Part print with two shaded views. Sizes in mm from the minimum x, y, z corner. A direction names the side the tool comes from. Round coordinates to 2 decimals unless told otherwise and drop trailing zeros. Order: outer loops, then holes, each group sorted by start corner. A loop starts at its lowest first (then second) coordinate and runs counter-clockwise, first axis right, second up. Notation, with made-up numbers: (8.25, -39) -> (30.25, -39) arc R30 ccw to (30.25, -15) -> close; hole circle Ø4 at (85.5, 72). An arc over 180 degrees is marked (long way). Use a Markdown table: item, result. Add a question column.
Item 1: Probe L1, parallel to X at y = 4.2, z = 8; L2, parallel to X at y = 3.4, z = 12.25; L3, parallel to Z at x = 18.25, y = 4.05. List the from-to ranges inside material, lowest first.
Item 2: Slice it at D-D, the plane x = 13.75. Give the cut face in (y, z), plus the area to 3 significant figures.
Item 3: Slice it at B-B, the plane y = 1.45. Give the cut face in (x, z).
Item 4: 3-axis set-ups, long thin cutter, end or side, ignore diameter. For the marked faces 5, 6, 7 and 8: which of +Z, -Z, +X, -X, +Y, -Y reach the whole face in a straight line?
Item 5: Slice it at C-C, the plane z = 7.25. Give the cut face in (x, y).
Item 6: Pin check, flat tips, straight feed: pin 1 (2 mm diameter, centred on x = 17.5, y = 1.5, fed in from -Z); pin 2 (1.5 mm diameter, centred on y = 3, z = 7, fed in from -X). Stop position of each tip, or through.
Item 7: Two-plate mould, pull along X, no slides. Class the marked faces 1, 2, 3 and 4: released by +X, released by -X, zero draft, split by the parting line, or undercut.
Item 8: Slice it at A-A, the plane z = 9.5. Give the cut face in (x, y).
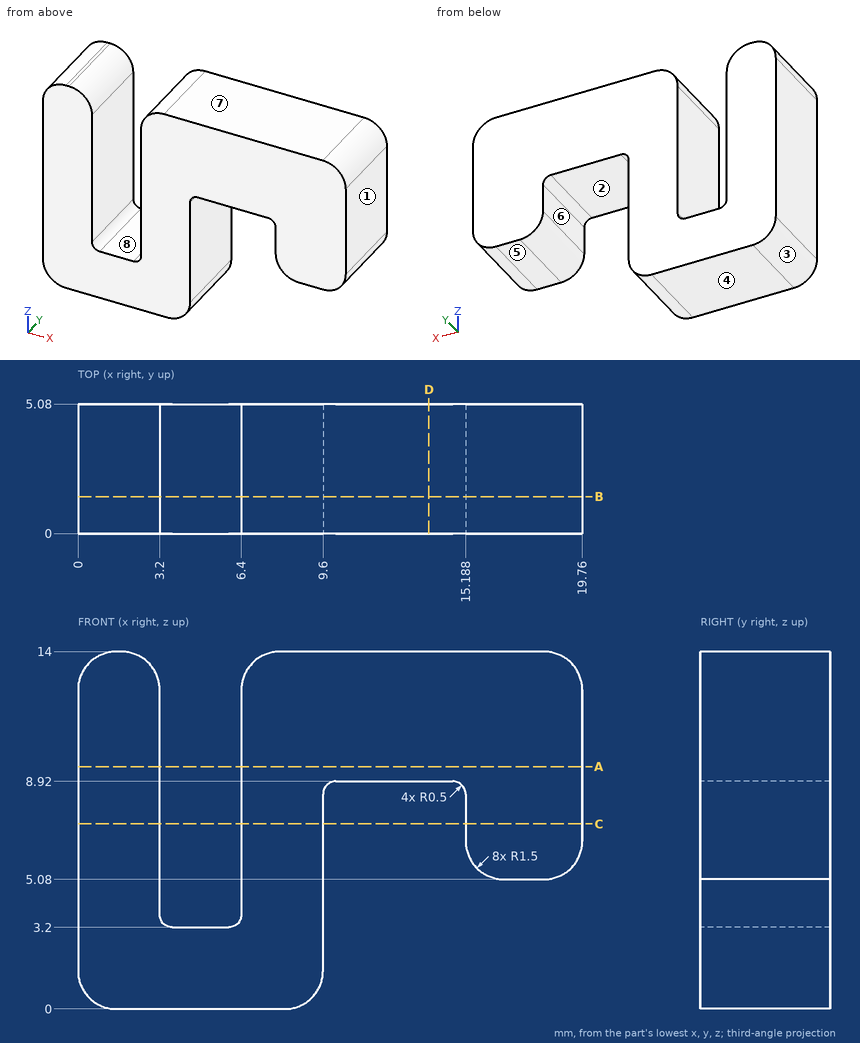
Check sheet entries:
| question | item | result |
|---|---|---|
| 1 | L1 | 0 to 3.2, 6.4 to 9.6, 15.19 to 19.76 |
| 1 | L2 | 0 to 3.2, 6.4 to 19.76 |
| 1 | L3 | 5.08 to 14 |
| 2 | outline | (0, 8.92) -> (5.08, 8.92) -> (5.08, 14) -> (0, 14) -> close |
| 2 | area | 25.8 mm2 |
| 3 | outline | (0, 1.5) arc R1.5 ccw to (1.5, 0) -> (8.1, 0) arc R1.5 ccw to (9.6, 1.5) -> (9.6, 8.42) arc R0.5 cw to (10.1, 8.92) -> (14.69, 8.92) arc R0.5 cw to (15.19, 8.42) -> (15.19, 6.58) arc R1.5 ccw to (16.69, 5.08) -> (18.26, 5.08) arc R1.5 ccw to (19.76, 6.58) -> (19.76, 12.5) arc R1.5 ccw to (18.26, 14) -> (7.9, 14) arc R1.5 ccw to (6.4, 12.5) -> (6.4, 3.7) arc R0.5 cw to (5.9, 3.2) -> (3.7, 3.2) arc R0.5 cw to (3.2, 3.7) -> (3.2, 12.5) arc R1.5 ccw to (1.7, 14) -> (1.5, 14) arc R1.5 ccw to (0, 12.5) -> close |
| 4 | face 5 | -Z, +X, +Y, -Y |
| 4 | face 6 | -Z, +Y, -Y |
| 4 | face 7 | +Z, +X, -X, +Y, -Y |
| 4 | face 8 | +Z, +Y, -Y |
| 5 | outline | (0, 0) -> (3.2, 0) -> (3.2, 5.08) -> (0, 5.08) -> close; (6.4, 0) -> (9.6, 0) -> (9.6, 5.08) -> (6.4, 5.08) -> close; (15.19, 0) -> (19.76, 0) -> (19.76, 5.08) -> (15.19, 5.08) -> close |
| 6 | pin 1 | z = 5.08 |
| 6 | pin 2 | x = 0 |
| 7 | face 1 | released by +X |
| 7 | face 2 | undercut |
| 7 | face 3 | released by -X |
| 7 | face 4 | zero draft |
| 8 | outline | (0, 0) -> (3.2, 0) -> (3.2, 5.08) -> (0, 5.08) -> close; (6.4, 0) -> (19.76, 0) -> (19.76, 5.08) -> (6.4, 5.08) -> close |
